Here's the drawing with two shaded views (mm, measured from the low corner). I have some questions. A direction names the side the tool comes from. Give positions to 0.01 mm unless a question says otherwise; leave off trailing zeros. Loops run counter-clockwise (first coordinate to the right, second up) from the corner with the lowest first, then second, coordinate; pieces in that order, holes last. Notation, with made-up numbers: (84.25, 15.25) -> (133.25, 15.25) arc R25 cw to (133.25, 51.25) -> close; hole circle Ø11 at (31.5, -10.75). An arc over 180 degrees is marked (long way). Answer in a Markdown table with one row per item. Add a question column.
Item 1: If we section it at B-B (z = 17): Write out the boundary of the cut face in (x, y), then the cut area to 3 significant figures.
Item 2: We'd pull the mould along Y, two halves only. Please class the marked faces 4, 5 and 6: released by +Y, released by -Y, zero draft, split by the parting line, or undercut.
Item 3: If we section it at D-D (y = 5): Write out the boundary of the cut face in (x, z).
Item 4: If I drill on line 1 (Y direction, x = 47, z = 35); line 2 (X direction, y = 4.75, z = 17); line 3 (X direction, y = 6.75, z = 12), over which ranges is the centre line in solid material (lowest first)?
Item 5: Which directions (+Z, -Z, +X, -X, +Y, -Y) give clear straight access to the entire face, cutting with the end or side of a thin tool? Please do the marked faces 1, 2 and 3.
Item 6: If we section it at C-C (x = 26.5): Write out the boundary of the cut face in (y, z).
Item 7: If we section it at A-A (y = 10.25): Write out the boundary of the cut face in (x, z).
Item 8: For P1, Ø20.5, axis at x = 26.5, z = 17, coming from the +Y side; P2, Ø10, axis at x = 17, z = 21.5, coming from the -Y side; P3, Ø1.5, axis at y = 9, z = 6, coming from the -X side; P4, Ø7, axis at x = 6, y = 6, coming from the -Z side, each with a flat end and sliding along its axis, tell me the tip position at first contact or that it passes through.
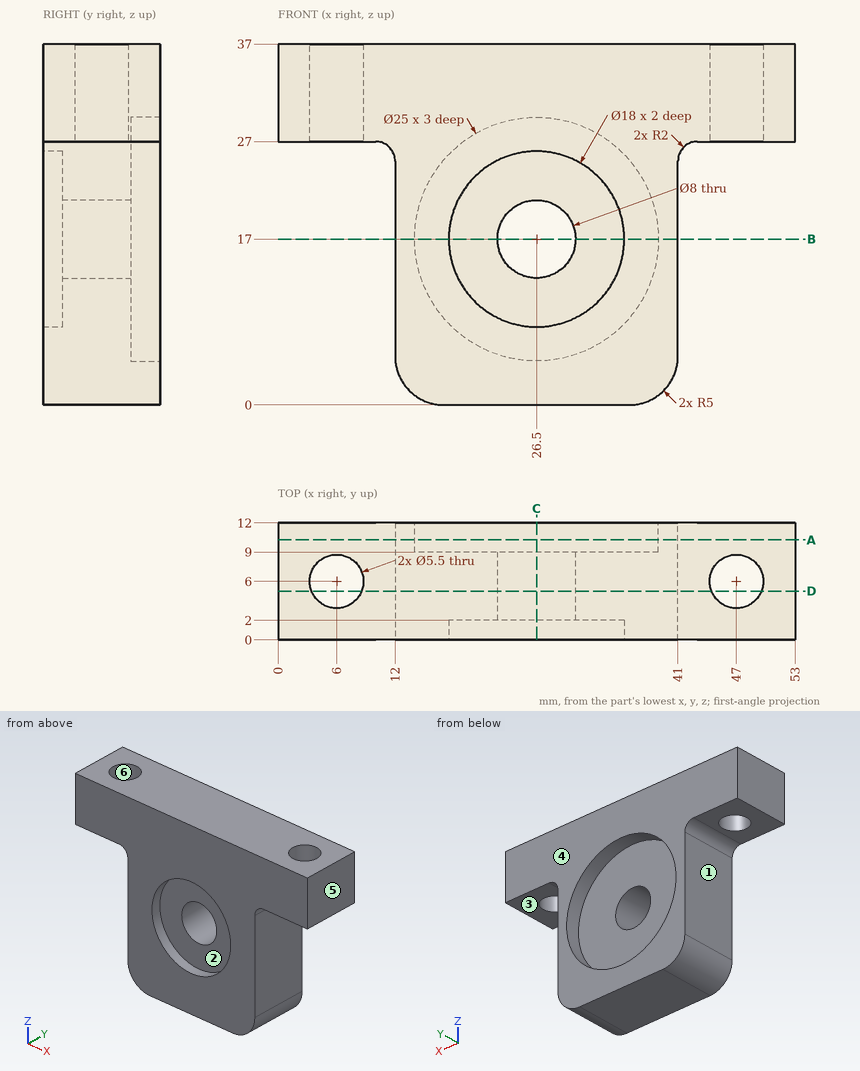
Recorded:
| question | item | result |
|---|---|---|
| 1 | outline | (12, 0) -> (17.5, 0) -> (17.5, 2) -> (22.5, 2) -> (22.5, 9) -> (14, 9) -> (14, 12) -> (12, 12) -> close; (30.5, 2) -> (35.5, 2) -> (35.5, 0) -> (41, 0) -> (41, 12) -> (39, 12) -> (39, 9) -> (30.5, 9) -> close |
| 1 | area | 181 mm^2 |
| 2 | face 4 | released by +Y |
| 2 | face 5 | zero draft |
| 2 | face 6 | undercut |
| 3 | outline | (0, 27) -> (3.44, 27) -> (3.44, 37) -> (0, 37) -> close; (8.56, 27) -> (10, 27) arc R2 cw to (12, 25) -> (12, 5) arc R5 ccw to (17, 0) -> (36, 0) arc R5 ccw to (41, 5) -> (41, 25) arc R2 cw to (43, 27) -> (44.44, 27) -> (44.44, 37) -> (8.56, 37) -> close; (49.56, 27) -> (53, 27) -> (53, 37) -> (49.56, 37) -> close; hole circle Ø8 at (26.5, 17) |
| 4 | line 1 | y = 0 to 3.25, 8.75 to 12 |
| 4 | line 2 | x = 12 to 22.5, 30.5 to 41 |
| 4 | line 3 | x = 12 to 41 |
| 5 | face 1 | -Z, -X, +Y, -Y |
| 5 | face 2 | -Y |
| 5 | face 3 | -Z, +X, +Y, -Y |
| 6 | outline | (0, 0) -> (12, 0) -> (12, 4.5) -> (9, 4.5) -> (9, 13) -> (2, 13) -> (2, 8) -> (0, 8) -> close; (0, 26) -> (2, 26) -> (2, 21) -> (9, 21) -> (9, 29.5) -> (12, 29.5) -> (12, 37) -> (0, 37) -> close |
| 7 | outline | (0, 27) -> (10, 27) arc R2 cw to (12, 25) -> (12, 5) arc R5 ccw to (17, 0) -> (36, 0) arc R5 ccw to (41, 5) -> (41, 25) arc R2 cw to (43, 27) -> (53, 27) -> (53, 37) -> (0, 37) -> close; hole circle Ø25 at (26.5, 17) |
| 8 | P1 | stops at y = 9 |
| 8 | P2 | stops at y = 0 |
| 8 | P3 | stops at x = 12 |
| 8 | P4 | stops at z = 27 |
